```python
from build123d import *

# Parameters (mm, degrees)
SKETCH1_W            = 74
SKETCH1_H            = 13
BOSS_EXTRUDE1_DEPTH  = 1.6
SKETCH2_W            = 74
SKETCH2_H            = 3
BOSS_EXTRUDE2_DEPTH  = 5.3
FILLET1_R            = 1
M2_CLEARANCE_HOLE1_D = 2.4


with BuildPart() as part:
    # Sketch1 → Boss-Extrude1 (new body)
    with BuildSketch(Plane(origin=(0, 0, 0), x_dir=(1, 0, 0), z_dir=(0, 1, 0))):
        Rectangle(SKETCH1_W, SKETCH1_H)
    extrude(amount=BOSS_EXTRUDE1_DEPTH)

    # Sketch2 → Boss-Extrude2 (add)
    with BuildSketch(Plane(origin=(0, 1.6, 0), x_dir=(1, 0, 0), z_dir=(0, 1, 0))):
        with Locations((0, 5)):
            Rectangle(SKETCH2_W, SKETCH2_H)
    extrude(amount=BOSS_EXTRUDE2_DEPTH)

    # Fillet1
    fillet1_edges = [part.edges().sort_by_distance(p)[0] for p in [
        (0, 1.6, -3.5),
    ]]
    fillet(fillet1_edges, radius=FILLET1_R)

    # M2 Clearance Hole1 (through all)
    with Locations(Plane(origin=(-22, 4.6, -6.5), x_dir=(-1, 0, 0), z_dir=(0, 0, -1))):
        with Locations((0, 0), (-22, 0), (-44, 0)):
            Hole(M2_CLEARANCE_HOLE1_D / 2)


solid = part.part
```
The model under review builds one solid part; all positions refer to its coordinate system, in mm. A direction names the side the tool comes from. Round coordinates to 2 decimals unless told otherwise and drop trailing zeros. Loops run counter-clockwise (first coordinate to the right, second up) from the corner with the lowest first, then second, coordinate; pieces in that order, holes last. Notation, with made-up numbers: (-13, 72.5) -> (3, 72.5) arc R15 cw to (3, 95.5) -> close; hole circle Ø4 at (80, 10). An arc over 180 degrees is marked (long way). Answer in a Markdown table with one row per item.
1) Consider section D-D, the plane x = -18.5. Write out the cut boundary in (y, z).
Taken from the geometry:
| item | result |
|---|---|
| outline | (0, -6.5) -> (6.9, -6.5) -> (6.9, -3.5) -> (2.6, -3.5) arc R1 cw to (1.6, -2.5) -> (1.6, 6.5) -> (0, 6.5) -> close |
2) For pin 1 Ø1.4 at (x, y) = (-22, 4.6) entering from +Z; pin 2 Ø2 at (x, z) = (2, -1.5) entering from +Y; pin 3 Ø1.3 at (x, y) = (5, 4) entering from +Z, all flat-tipped, find the tip position at first contact; note any pin that passes through.
Taken from the geometry:
| item | result |
|---|---|
| pin 1 | passes through |
| pin 2 | stops at y = 1.6 |
| pin 3 | stops at z = -3.5 |
3) Tool access review of faces 5 (the flat face through (-37, 1, -3)), 6 (the flat face through (-1, 3, -3.5)): name each direction out of +Z, -Z, +X, -X, +Y, -Y from which nothing blocks a thin tool from reaching the whole face with its end or side.
Taken from the geometry:
| item | result |
|---|---|
| face 5 | +Z, -Z, -X, +Y, -Y |
| face 6 | +Z, +X, -X, +Y |
4) Consider section C-C, the plane y = 4.6. Write out the cut boundary in (x, z).
Taken from the geometry:
| item | result |
|---|---|
| outline | (-37, -6.5) -> (-23.2, -6.5) -> (-23.2, -3.5) -> (-37, -3.5) -> close; (-20.8, -6.5) -> (-1.2, -6.5) -> (-1.2, -3.5) -> (-20.8, -3.5) -> close; (1.2, -6.5) -> (20.8, -6.5) -> (20.8, -3.5) -> (1.2, -3.5) -> close; (23.2, -6.5) -> (37, -6.5) -> (37, -3.5) -> (23.2, -3.5) -> close |
5) Consider section A-A, the plane x = 0. Write out the cut boundary in (y, z).
Taken from the geometry:
| item | result |
|---|---|
| outline | (0, -6.5) -> (3.4, -6.5) -> (3.4, -3.5) -> (2.6, -3.5) arc R1 cw to (1.6, -2.5) -> (1.6, 6.5) -> (0, 6.5) -> close; (5.8, -6.5) -> (6.9, -6.5) -> (6.9, -3.5) -> (5.8, -3.5) -> close |
6) Wall thickness on line 1 along Y through (x, z) = (-22, -5.9); line 2 along Z through (x, y) = (18, 2.5); line 3 along Y through (x, z) = (20, 4.5): over which ranges is each line inside the solid? List them lowest first.
Taken from the geometry:
| item | result |
|---|---|
| line 1 | y = 0 to 3.4, 5.8 to 6.9 |
| line 2 | z = -6.5 to -3.49 |
| line 3 | y = 0 to 1.6 |
7) Draft analysis for pull direction Y (two halves, no side actions). For faces 1 (the flat face through (-1, 3, -6.5)), 2 (the flat face through (-1, 0, 0)), 3 (the flat face through (-1, 1.6, 2)), 4 (the cylindrical face through (-22.95, 3.87, -4.98)), state which applies: pulls with the +Y half, pulls with the -Y half, needs draft (parallel to the pull), parting line crosses it, or undercut.
Taken from the geometry:
| item | result |
|---|---|
| face 1 | needs draft |
| face 2 | pulls with the -Y half |
| face 3 | pulls with the +Y half |
| face 4 | undercut |
8) Consider section B-B, the plane z = -5.25. Write out the cut boundary in (x, y), plus the area to 3 significant figures.
Taken from the geometry:
| item | result |
|---|---|
| outline | (-37, 0) -> (37, 0) -> (37, 6.9) -> (-37, 6.9) -> close; hole circle Ø2.4 at (-22, 4.6); hole circle Ø2.4 at (0, 4.6); hole circle Ø2.4 at (22, 4.6) |
| area | 497 mm² |
